For this review, take the finished solid that the model builds, in its own axes (mm). Face numbers are marked on the shaded views. A direction names the side the tool comes from. Coordinates: 2 decimals unless noted, no trailing zeros. Loops run counter-clockwise (first coordinate to the right, second up) from the corner with the lowest first, then second, coordinate; pieces in that order, holes last.
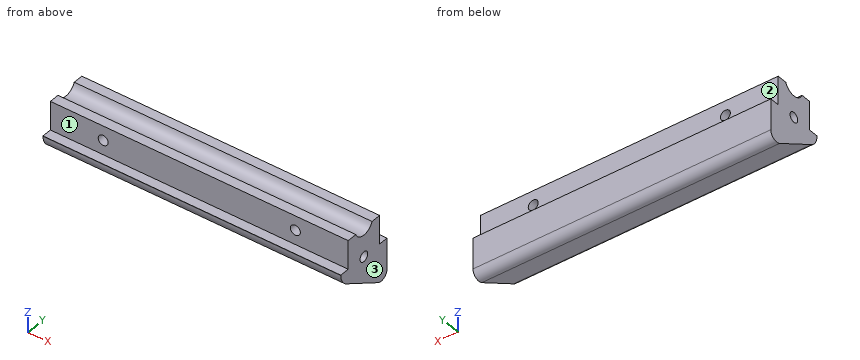
```python
from build123d import *

# Parameters (mm, degrees)
BOSS_EXTRUDE1_DEPTH = 98.425
CUT_EXTRUDE2_DEPTH  = 98.425
SKETCH5_R           = 1.651
CUT_EXTRUDE3_DEPTH  = 13.5992
FILLET1_R           = 2.54
SKETCH6_R           = 1.651
CUT_EXTRUDE4_DEPTH  = 98.425


with BuildPart() as part:
    # Sketch1 → Boss-Extrude1 (new body)
    with BuildSketch(Plane(origin=(0, 0, 0), x_dir=(0, 0, -1), z_dir=(1, 0, 0))):
        with BuildLine():
            Line((0, 16.7996), (0, 3.2004))
            Line((0, 3.2004), (9.525, 3.2004))
            Line((9.525, 3.2004), (9.525, 0))
            Line((9.525, 0), (9.672001208, 0))
            ThreePointArc((9.672001208, 0), (12.1043061, 0.647018058), (13.89365381, 2.417039025))
            Line((13.89365381, 2.417039025), (24.215623453, 20))
            Line((24.215623453, 20), (9.525, 20))
            Line((9.525, 20), (9.525, 16.7996))
            Line((9.525, 16.7996), (0, 16.7996))
        make_face()
    extrude(amount=BOSS_EXTRUDE1_DEPTH)

    # Sketch4 → Cut-Extrude2 (cut)
    with BuildSketch(Plane.ZY):
        with BuildLine():
            Line((0, 13.526281186), (0, 6.473718814))
            ThreePointArc((0, 6.473718814), (-2.36728, 10), (0, 13.526281186))
        make_face()
    extrude(amount=-CUT_EXTRUDE2_DEPTH, mode=Mode.SUBTRACT)

    # Sketch5 → Cut-Extrude3 (cut)
    with BuildSketch(Plane(origin=(0, 16.7996, 0), x_dir=(1, 0, 0), z_dir=(0, 1, 0))):
        with Locations((17.4625, 4.7625)):
            Circle(SKETCH5_R)
        with Locations((80.9625, 4.7625)):
            Circle(SKETCH5_R)
    extrude(amount=-CUT_EXTRUDE3_DEPTH, mode=Mode.SUBTRACT)

    # Fillet1
    fillet1_edges = [part.edges().sort_by_distance(p)[0] for p in [
        (49.2125, 20, -24.215623453),
    ]]
    fillet(fillet1_edges, radius=FILLET1_R)

    # Sketch6 → Cut-Extrude4 (cut)
    with BuildSketch(Plane(origin=(98.425, 0, 0), x_dir=(0, 0, -1), z_dir=(1, 0, 0))):
        with Locations((9.525, 10)):
            Circle(SKETCH6_R)
    extrude(amount=-CUT_EXTRUDE4_DEPTH, mode=Mode.SUBTRACT)


solid = part.part
```
Q1. Consider section A-A (y = 10). State the section outline as (x, z) points (1 decimal).
Q2. Machinability: for the marked faces 1, 2 and 3, which of the approach directions +Z, -Z, +X, -X, +Y, -Y give a long, thin tool a straight path to every point of the face, cutting with its end or side? Answer none if there is none.
Q3. Consider section B-B (x = 6.5). State the section outline as (y, z) points (3 decimals), then the cut area to 3 significant figures.
Q4. For pin 1 Ø4 at (x, z) = (80.96, -4.76) entering from +Y; pin 2 Ø1 at (x, z) = (75, -5) entering from -Y; pin 3 Ø2.5 at (x, z) = (17.46, -4.76) entering from +Y; pin 4 Ø12 at (x, y) = (36.5, 9.5) entering from -Z, all flat-tipped, find the tip position at first contact; note any pin that passes through.
Q5. Wall thickness on probe 1 along Y at (x, z) = (91, -2); probe 2 along Y at (x, z) = (79, -2.75); probe 3 along Y at (x, z) = (9.5, -8.25): over which ranges is each line inside the solid? List them lowest first.
Q6. Consider section D-D (z = -16.5). State the section outline as (x, y) points (3 decimals).
Q7. Consider section C-C (y = 4.25). State the section outline as (x, z) points (1 decimal).
Model answer:
1. outline: (0, -18.3) - (98.4, -18.3) - (98.4, -11.2) - (0, -11.2) - close; (0, -7.9) - (98.4, -7.9) - (98.4, -2.4) - (0, -2.4) - close; hole circle Ø3.3 at (17.5, -4.8); hole circle Ø3.3 at (81, -4.8)
2. face 1: +Z, +X, -X, -Y
2. face 2: +Z, +X, -X, +Y
2. face 3: +Z, -Z, +X, +Y, -Y
3. outline: (0, -9.672) arc R4.895 ccw to (2.417, -13.894) - (16.174, -21.97) arc R2.54 ccw to (20, -19.779) - (20, -9.525) - (16.8, -9.525) - (16.8, 0) - (13.526, 0) arc R3.81 cw to (6.474, 0) - (3.2, 0) - (3.2, -9.525) - (0, -9.525) - close; hole circle Ø3.302 at (10, -9.525)
3. area: 280 mm2
4. pin 1: stops at y = 16.8
4. pin 2: stops at y = 3.2
4. pin 3: passes through
4. pin 4: stops at z = -21.57
5. probe 1: y = 3.2 to 8.37, 11.63 to 16.8
5. probe 2: y = 3.2 to 16.8
5. probe 3: y = 3.2 to 8.95, 11.05 to 16.8
6. outline: (0, 6.857) - (98.425, 6.857) - (98.425, 20) - (0, 20) - close
7. outline: (0, -15) - (98.4, -15) - (98.4, 0) - (0, 0) - close; hole circle Ø3.3 at (17.5, -4.8); hole circle Ø3.3 at (81, -4.8)
